Could you check a few things on this model? Use its own coordinates, in mm. Face numbers are marked on the shaded views. A direction names the side the tool comes from. Coordinates: 2 decimals unless noted, no trailing zeros. Loops run counter-clockwise (first coordinate to the right, second up) from the corner with the lowest first, then second, coordinate; pieces in that order, holes last. Notation, with made-up numbers: (12.25, -17) -> (43.25, -17) arc R15 cw to (43.25, -9) -> close; hole circle Ø4 at (1.25, 10.25). An arc over 180 degrees is marked (long way). One line per question, with ' | ' between items.
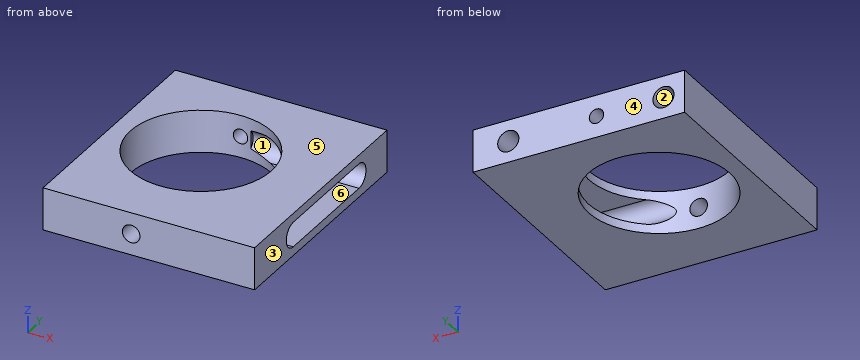
from build123d import *

# Parameters (mm, degrees)
SKETCH1_W                     = 35
SKETCH1_H                     = 33.23
SKETCH1_R                     = 10
BOSS_EXTRUDE1_DEPTH           = 6
CUT_EXTRUDE1_DEPTH            = 16
F_3_0MM_DOWEL_HOLE1_D         = 3
F_3_0MM_DOWEL_HOLE1_DEPTH     = 7.2
F_3_0MM_DOWEL_HOLE1_TIP       = 0.901290929
SKETCH9_W                     = 6
SKETCH9_H                     = 33.23
CUT_EXTRUDE2_DEPTH            = 5
M2_5X0_45_TAPPED_HOLE1_REACH  = 40.033
M2_5X0_45_TAPPED_HOLE1_BORE_R = 1.025
M3X0_5_TAPPED_HOLE2_REACH     = 40.033
M3X0_5_TAPPED_HOLE2_BORE_R    = 1.25


with BuildPart() as part:
    # Sketch1 → Boss-Extrude1 (new body)
    with BuildSketch(Plane.XY):
        with Locations((0, -0.885)):
            Rectangle(SKETCH1_W, SKETCH1_H)
        Circle(SKETCH1_R, mode=Mode.SUBTRACT)
    extrude(amount=BOSS_EXTRUDE1_DEPTH)

    # Sketch2 → Cut-Extrude1 (cut)
    with BuildSketch(Plane(origin=(17.5, 0, 0), x_dir=(0, 0, -1), z_dir=(1, 0, 0))):
        with BuildLine():
            Line((-4.75, -7.806071268), (-4.75, 8.693928732))
            ThreePointArc((-4.75, 8.693928732), (-3, 10.443928732), (-1.25, 8.693928732))
            Line((-1.25, 8.693928732), (-1.25, -7.806071268))
            ThreePointArc((-1.25, -7.806071268), (-3, -9.556071268), (-4.75, -7.806071268))
        make_face()
    extrude(amount=-CUT_EXTRUDE1_DEPTH, mode=Mode.SUBTRACT)

    # Ø3.0mm Dowel Hole1
    with Locations(Plane(origin=(0, 15.73, 0), x_dir=(1, 0, 0), z_dir=(0, 1, 0))):
        with Locations((-9.5, -3), (12.5, -3)):
            Hole(F_3_0MM_DOWEL_HOLE1_D / 2, depth=F_3_0MM_DOWEL_HOLE1_DEPTH)
            with Locations((0, 0, -(F_3_0MM_DOWEL_HOLE1_DEPTH + F_3_0MM_DOWEL_HOLE1_TIP / 2))):  # 118° drill point
                Cone(0, F_3_0MM_DOWEL_HOLE1_D / 2, F_3_0MM_DOWEL_HOLE1_TIP, mode=Mode.SUBTRACT)

    # Sketch9 → Cut-Extrude2 (cut)
    with BuildSketch(Plane.ZY.offset(17.5)):
        with Locations((3, -0.885)):
            Rectangle(SKETCH9_W, SKETCH9_H)
    extrude(amount=-CUT_EXTRUDE2_DEPTH, mode=Mode.SUBTRACT)

    # M2.5x0.45 Tapped Hole1 bore → M2.5x0.45 Tapped Hole1 (cut, up to next)
    with BuildSketch(Plane(origin=(0, 15.73, 0), x_dir=(1, 0, 0), z_dir=(0, 1, 0)), mode=Mode.PRIVATE) as m2_5x0_45_tapped_hole1_sk1:
        with Locations((0, -3)):
            Circle(M2_5X0_45_TAPPED_HOLE1_BORE_R)
    m2_5x0_45_tapped_hole1_tool1 = extrude(m2_5x0_45_tapped_hole1_sk1.sketch, amount=-M2_5X0_45_TAPPED_HOLE1_REACH, mode=Mode.PRIVATE) & part.part
    add(m2_5x0_45_tapped_hole1_tool1.solids().sort_by_distance((0, 15.73, 3))[0], mode=Mode.SUBTRACT)

    # M3x0.5 Tapped Hole2 bore → M3x0.5 Tapped Hole2 (cut, up to next)
    with BuildSketch(Plane(origin=(0, -17.5, 0), x_dir=(-1, 0, 0), z_dir=(0, -1, 0)), mode=Mode.PRIVATE) as m3x0_5_tapped_hole2_sk1:
        with Locations((0, -2.990437558)):
            Circle(M3X0_5_TAPPED_HOLE2_BORE_R)
    m3x0_5_tapped_hole2_tool1 = extrude(m3x0_5_tapped_hole2_sk1.sketch, amount=-M3X0_5_TAPPED_HOLE2_REACH, mode=Mode.PRIVATE) & part.part
    add(m3x0_5_tapped_hole2_tool1.solids().sort_by_distance((0, -17.5, 2.990438))[0], mode=Mode.SUBTRACT)


solid = part.part
1) If we section it at A-A on y = 0: Please give me the cut outline in (x, z), and give its area (4 significant figures).
Data:
outline: (-12.5, 0) -> (-10, 0) -> (-10, 6) -> (-12.5, 6) -> close; (10, 0) -> (17.5, 0) -> (17.5, 1.25) -> (10, 1.25) -> close; (10, 4.75) -> (17.5, 4.75) -> (17.5, 6) -> (10, 6) -> close | area: 33.75 mm²
2) If we section it at B-B on x = 0: Please give me the cut outline in (y, z) (3 decimals).
Data:
outline: (-17.5, 0) -> (-10, 0) -> (-10, 1.74) -> (-17.5, 1.74) -> close; (-17.5, 4.24) -> (-10, 4.24) -> (-10, 6) -> (-17.5, 6) -> close; (10, 0) -> (15.73, 0) -> (15.73, 1.975) -> (10, 1.975) -> close; (10, 4.025) -> (15.73, 4.025) -> (15.73, 6) -> (10, 6) -> close
3) I need wall thicknesses on line 1 along Z through (x, y) = (6.5, 8); line 2 along Z through (x, y) = (0, 14) (3 decimals); line 3 along X through (y, z) = (-8.5, 5.75). Which ranges of each line are inside material? Lowest first, please. Write a range as from..to.
Data:
line 1: 0..1.25, 4.75..6 | line 2: 0..1.975, 4.025..6 | line 3: -12.5..-5.27, 5.27..17.5
4) I'm going to push flat-ended pins straight in: pin 1 Ø2.5 at (x, z) = (12.5, 3) entering from +Y; pin 2 Ø10 at (x, y) = (11.5, -3) entering from -Z. Where does each tip first touch, or does it pass through?
Data:
pin 1: y = -9.03 | pin 2: z = 0
5) We'd pull the mould along Z, two halves only. Please class the marked faces 4, 5 and 6: pulls with the +Z half, pulls with the -Z half, needs draft (parallel to the pull), parting line crosses it, or undercut.
Data:
face 4: needs draft | face 5: pulls with the +Z half | face 6: undercut
6) On a 3-axis mill with a long thin cutter (end or side, diameter ignored), from which of +Z, -Z, +X, -X, +Y, -Y can I reach the whole of each face in a straight line? I mean the marked faces 1, 2 and 3. Say none if no direction works.
Data:
face 1: +X | face 2: +Y | face 3: +Z, -Z, +X, +Y, -Y
7) If we section it at D-D on x = 12.5: Please give me the cut outline in (y, z).
Data:
outline: (-17.5, 0) -> (15.73, 0) -> (15.73, 1.5) -> (9.6, 1.5) arc R1.75 cw to (8.69, 1.25) -> (-7.81, 1.25) arc R1.75 cw to (-7.81, 4.75) -> (8.69, 4.75) arc R1.75 cw to (9.6, 4.5) -> (15.73, 4.5) -> (15.73, 6) -> (-17.5, 6) -> close
8) If we section it at C-C on y = 13.5: Please give me the cut outline in (x, z) (3 decimals), and give its area (3 significant figures).
Data:
outline: (-12.5, 0) -> (17.5, 0) -> (17.5, 6) -> (-12.5, 6) -> close; hole circle Ø3 at (-9.5, 3); hole circle Ø2.05 at (0, 3); hole circle Ø3 at (12.5, 3) | area: 163 mm²
